The listing builds one solid part. Answer for the finished solid, in the listing's coordinates (mm). Coordinates: 2 decimals unless noted, no trailing zeros. Write each loop counter-clockwise with the first axis right and the second up, starting at its lowest first coordinate (ties: lowest second). Pieces come first, ordered by that corner, then holes.
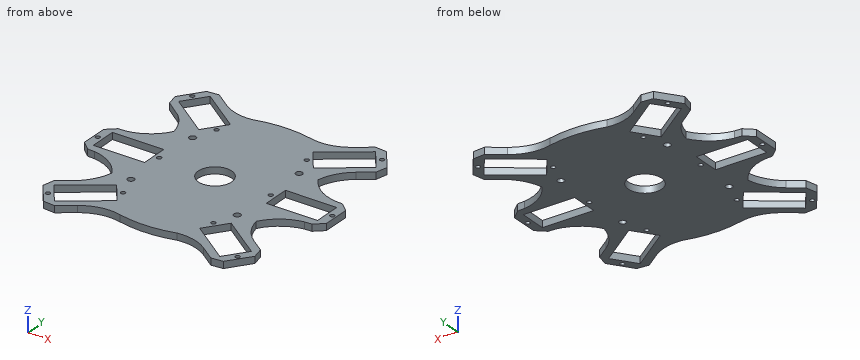
```python
from build123d import *

# Parameters (mm, degrees)
BOSS_EXTRUDE1_DEPTH = 3
SKETCH2_W           = 23
SKETCH2_H           = 12.24
CUT_EXTRUDE1_DEPTH  = 3
SKETCH3_R           = 7.46
SKETCH3_R_2         = 1
CUT_EXTRUDE2_DEPTH  = 3
SKETCH4_R           = 1.5
CUT_EXTRUDE4_DEPTH  = 3


with BuildPart() as part:
    # Sketch1 → Boss-Extrude1 (new body)
    with BuildSketch(Plane.XY):
        with BuildLine():
            Line((82.647113629, 154.567509506), (89.844393112, 164.473715786))
            Line((89.844393112, 164.473715786), (95.137710251, 164.954136674))
            Line((95.137710251, 164.954136674), (101.943215616, 160.009648062))
            ThreePointArc((101.943215616, 160.009648062), (108.747642501, 156.812557566), (116.251704746, 156.353577499))
            ThreePointArc((116.251704746, 156.353577499), (128.935389479, 158.162930803), (141.678042243, 156.830857858))
            ThreePointArc((141.678042243, 156.830857858), (150.42338057, 156.539561763), (158.456083243, 160.009645858))
            Line((158.456083243, 160.009645858), (165.261591353, 164.954136376))
            Line((165.261591353, 164.954136376), (170.55490849, 164.473715466))
            Line((170.55490849, 164.473715466), (177.752187889, 154.567509125))
            Line((177.752187889, 154.567509125), (176.573368159, 149.384810766))
            Line((176.573368159, 149.384810766), (170.515619404, 144.983599161))
            ThreePointArc((170.515619404, 144.983599161), (165.346551478, 139.353755533), (162.56771378, 132.23389152))
            ThreePointArc((162.56771378, 132.23389152), (168.807132787, 125.625610798), (177.296006603, 122.379267473))
            Line((177.296006603, 122.379267473), (180.529625637, 122.208660353))
            Line((180.529625637, 122.208660353), (184.529626293, 118.70866071))
            Line((184.529626293, 118.70866071), (184.529626293, 106.463914621))
            Line((184.529626293, 106.463914621), (180.529628861, 102.963911295))
            Line((180.529628861, 102.963911295), (177.296136644, 102.79331796))
            ThreePointArc((177.296136644, 102.79331796), (168.816865326, 99.532528302), (162.567726238, 92.938663582))
            ThreePointArc((162.567726238, 92.938663582), (165.335032155, 85.811599743), (170.515615031, 80.188915148))
            Line((170.515615031, 80.188915148), (176.573365794, 75.787706307))
            Line((176.573365794, 75.787706307), (177.752187889, 70.605008486))
            Line((177.752187889, 70.605008486), (170.55491301, 60.698798861))
            Line((170.55491301, 60.698798861), (165.261596092, 60.218375535))
            Line((165.261596092, 60.218375535), (158.456093799, 65.162857082))
            ThreePointArc((158.456093799, 65.162857082), (151.641647942, 68.320751195), (144.1475976, 68.818924897))
            ThreePointArc((144.1475976, 68.818924897), (131.464672299, 66.969153974), (118.721260324, 68.341632719))
            ThreePointArc((118.721260324, 68.341632719), (109.975917376, 68.632921623), (101.943212729, 65.162831055))
            Line((101.943212729, 65.162831055), (95.13771499, 60.21834324))
            Line((95.13771499, 60.21834324), (89.844397632, 60.698761712))
            Line((89.844397632, 60.698761712), (82.647113629, 70.604964708))
            Line((82.647113629, 70.604964708), (83.825933315, 75.787663077))
            Line((83.825933315, 75.787663077), (89.883680023, 80.188877497))
            ThreePointArc((89.883680023, 80.188877497), (95.064494698, 85.811419139), (97.831557073, 92.938633252))
            ThreePointArc((97.831557073, 92.938633252), (91.592138066, 99.546913975), (83.10326425, 102.7932573))
            Line((83.10326425, 102.7932573), (79.869645216, 102.96386442))
            Line((79.869645216, 102.96386442), (75.86964456, 106.463864062))
            Line((75.86964456, 106.463864062), (75.86964456, 118.708610151))
            Line((75.86964456, 118.708610151), (79.869645216, 122.208609794))
            Line((79.869645216, 122.208609794), (83.10313759, 122.37920015))
            ThreePointArc((83.10313759, 122.37920015), (91.594370453, 125.622109158), (97.831557073, 132.233840961))
            ThreePointArc((97.831557073, 132.233840961), (95.706766675, 138.255067903), (91.855628915, 143.348067616))
            Line((91.855628915, 143.348067616), (83.825933315, 149.384811137))
            Line((83.825933315, 149.384811137), (82.647113629, 154.567509506))
        make_face()
    extrude(amount=BOSS_EXTRUDE1_DEPTH)

    # Sketch2 → Cut-Extrude1 (cut)
    with BuildSketch(Plane.XY.offset(3)):
        Polygon((85.883180637, 152.216369421), (93.077671686, 162.118737751), (111.685063156, 148.599677772), (104.490572106, 138.697309442), align=None)
        Polygon((111.684568391, 76.57424171), (104.489714954, 86.476346739), (85.883095664, 72.956224001), (93.077671686, 63.054500773), align=None)
        with Locations((91.369645216, 112.588609794)):
            Rectangle(SKETCH2_W, SKETCH2_H)
        Polygon((167.318839084, 162.122576423), (174.502849909, 152.212602231), (155.881166379, 138.713235486), (148.664694499, 148.599677772), align=None)
        with Locations((169.029625637, 112.588609794)):
            Rectangle(SKETCH2_W, SKETCH2_H)
        Polygon((174.516118852, 72.956145779), (167.3172806, 63.056937335), (148.715826824, 76.584166078), (155.914665077, 86.483374522), align=None)
    extrude(amount=-CUT_EXTRUDE1_DEPTH, mode=Mode.SUBTRACT)

    # Sketch3 → Cut-Extrude2 (cut)
    with BuildSketch(Plane.XY.offset(3)):
        with Locations((130.211941481, 112.566154055)):
            Circle(SKETCH3_R)
        with Locations((87.619687014, 158.519459583)):
            Circle(SKETCH3_R_2)
        with Locations((109.948556778, 142.296587609)):
            Circle(SKETCH3_R_2)
        with Locations((172.773012849, 158.517526001)):
            Circle(SKETCH3_R_2)
        with Locations((150.415193897, 142.300427521)):
            Circle(SKETCH3_R_2)
        with Locations((182.829625637, 112.588609794)):
            Circle(SKETCH3_R_2)
        with Locations((155.229625637, 112.588609794)):
            Circle(SKETCH3_R_2)
        with Locations((105.169645216, 112.588609794)):
            Circle(SKETCH3_R_2)
        with Locations((77.567644425, 112.588609794)):
            Circle(SKETCH3_R_2)
        with Locations((109.947817472, 82.877287408)):
            Circle(SKETCH3_R_2)
        with Locations((87.619707876, 66.653369203)):
            Circle(SKETCH3_R_2)
        with Locations((172.776845103, 66.653818683)):
            Circle(SKETCH3_R_2)
        with Locations((150.455100573, 82.886493174)):
            Circle(SKETCH3_R_2)
    extrude(amount=-CUT_EXTRUDE2_DEPTH, mode=Mode.SUBTRACT)

    # Sketch4 → Cut-Extrude4 (cut)
    with BuildSketch(Plane.XY.offset(3)):
        with Locations((106.267728038, 132.297669996)):
            Circle(SKETCH4_R)
        with Locations((154.06771378, 132.23389152)):
            Circle(SKETCH4_R)
        with Locations((106.331557073, 92.938633252)):
            Circle(SKETCH4_R)
        with Locations((154.067726238, 92.938663582)):
            Circle(SKETCH4_R)
    extrude(amount=-CUT_EXTRUDE4_DEPTH, mode=Mode.SUBTRACT)


solid = part.part
```
(1) Section C-C, the plane z = 0.6 is taken. State how many separate pieces and enclosed holes the cut face has, plus the area to 3 significant figures.
(2) Section B-B, the plane y = 137 is taken. Write down the section's boundary in (x, z).
(3) Section A-A, the plane x = 164 is taken. Write down the section's boundary in (y, z).
(4) Find the intervals of material crossed by probe 1 along Y at (x, z) = (180, 0.5); probe 2 along Y at (x, z) = (103.5, 1.45); probe 3 along X at (y, z) = (110, 2.8), in increasing order.
(5) Each of these flat-tipped pins is pushed along its axis until it touches: pin 1 (1.5 mm diameter, centred on x = 171.5, z = 1.5, fed in from +Y); pin 2 (1.5 mm diameter, centred on x = 170.5, z = 2, fed in from -Y). Where does it stop, or does it pass through?
Solution:
1. separate pieces: 1
1. enclosed holes: 23
1. area: 6,060 mm2
2. outline: (96.33, 0) - (164.08, 0) - (164.08, 3) - (96.33, 3) - close
3. outline: (61.13, 0) - (65.47, 0) - (65.47, 3) - (61.13, 3) - close; (80.6, 0) - (88.33, 0) - (88.33, 3) - (80.6, 3) - close; (95.04, 0) - (106.47, 0) - (106.47, 3) - (95.04, 3) - close; (118.71, 0) - (130.12, 0) - (130.12, 3) - (118.71, 3) - close; (136.82, 0) - (144.6, 0) - (144.6, 3) - (136.82, 3) - close; (159.72, 0) - (164.04, 0) - (164.04, 3) - (159.72, 3) - close
4. probe 1: y = 102.94 to 106.47, 118.71 to 122.24
4. probe 2: y = 66.19 to 70.63, 85.76 to 139.42, 154.55 to 158.99
4. probe 3: x = 75.87 to 79.87, 102.87 to 123.21, 137.22 to 157.53, 180.53 to 184.53
5. pin 1: stops at y = 164.21
5. pin 2: stops at y = 60.63
